Input: part model. Units: mm. Frame: model coordinates. A direction names the side the tool comes from. Give positions to 0.01 mm unless a question says otherwise; leave off trailing zeros. Loops run counter-clockwise (first coordinate to the right, second up) from the corner with the lowest first, then second, coordinate; pieces in that order, holes last. Notation, with made-up numbers: M 63,8 L 98,8 A19 ccw 98,17 Z; hole C 61,60 d6. An arc over 180 degrees is marked long. Use a Markdown table: item, result. Add a question column.
from build123d import *

# Parameters (mm, degrees)
BOSS_EXTRUDE1_DEPTH  = 6.35
SKETCH6_W            = 57.15
SKETCH6_H            = 4.7625
SKETCH6_W_2          = 15.875
CUT_EXTRUDE1_DEPTH   = 85.197384349
M5_CLEARANCE_HOLE1_D = 5.5


with BuildPart() as part:
    # Sketch2 → Boss-Extrude1 (new body)
    with BuildSketch(Plane(origin=(0, 0, 0), x_dir=(1, 0, 0), z_dir=(0, 1, 0))):
        with BuildLine():
            Line((0, 11.1125), (69.85, 11.1125))
            ThreePointArc((69.85, 11.1125), (80.9625, 0), (69.85, -11.1125))
            Line((69.85, -11.1125), (0, -11.1125))
            ThreePointArc((0, -11.1125), (-11.1125, 0), (0, 11.1125))
        make_face()
        with BuildLine():
            Line((15.875, 7.9375), (53.975, 7.9375))
            ThreePointArc((53.975, 7.9375), (61.9125, 0), (53.975, -7.9375))
            Line((53.975, -7.9375), (15.875, -7.9375))
            ThreePointArc((15.875, -7.9375), (7.9375, 0), (15.875, 7.9375))
        make_face(mode=Mode.SUBTRACT)
    extrude(amount=BOSS_EXTRUDE1_DEPTH)

    # Sketch6 → Cut-Extrude1 (cut, through all)
    with BuildSketch(Plane(origin=(0, 0, -11.1125), x_dir=(-1, 0, 0), z_dir=(0, 0, -1))):
        with Locations((-34.925, 2.38125)):
            Rectangle(SKETCH6_W, SKETCH6_H)
        with Locations((-73.025, 3.96875)):
            Rectangle(SKETCH6_W_2, SKETCH6_H)
        with Locations((3.175, 3.96875)):
            Rectangle(SKETCH6_W_2, SKETCH6_H)
    extrude(amount=-CUT_EXTRUDE1_DEPTH, mode=Mode.SUBTRACT)

    # M5 Clearance Hole1 (through all)
    with Locations(Plane(origin=(0, 1.5875, 0), x_dir=(1, 0, 0), z_dir=(0, 1, 0))):
        with Locations((-1.5875, 0), (71.4375, 0)):
            Hole(M5_CLEARANCE_HOLE1_D / 2)


solid = part.part
1) Section query A-A, the plane z = 0. Return the cut outline in (x, y).
2) Section query B-B, the plane y = 3. Return the cut outline in (x, z).
3) Section query D-D, the plane z = -5.75. Return the cut outline in (x, y), and give its area (3 significant figures).
4) Pull-direction query (X, two-part tool) for faces 5 (the cylindrical face through (7.94, 5.55, 0.17)), 6 (the flat face through (70, 0, -3)), 7 (the flat face through (65.088, 4, 0)), 8 (the flat face through (35, 6, 7.938)); classes: pulls with the +X half, pulls with the -X half, needs draft (parallel to the pull), parting line crosses it, or undercut.
5) Section query C-C, the plane x = 39. Return the cut outline in (y, z), and give its area (3 significant figures).
6) Contact query for flat-ended pins moving along their axis: P1, Ø1.4, axis at y = 5, z = 5.5, coming from the +X side; P2, Ø1.4, axis at y = 3, z = -4, coming from the -X side; P3, Ø5, axis at x = 1, z = -0.5, coming from the +Y side; P4, Ø10, axis at x = -0.5, z = 3, coming from the -Y side. Output: stop coordinate, or through.
7) Ray query, line 1 (Z direction, x = 38, y = 5.75); line 2 (X direction, y = 2.5, z = -1.25); line 3 (Y direction, x = 61.5, z = 7.75). Return the intervals inside material, ascending. Write a range as [from, to].
8) Reachability of faces 1 (the flat face through (63.5, 2, 0)), 2 (the cylindrical face through (61.91, 5.55, -0.17)), 3 (the flat face through (75, 1.588, 0)), 4 (the flat face through (4.762, 4, 0)) from +Z, -Z, +X, -X, +Y, -Y: full face, straight path, thin tool, end or side. Return the list, or none.
Entries:
| question | item | result |
|---|---|---|
| 1 | outline | M -11.11,0 L -4.34,0 L -4.34,1.59 L -11.11,1.59 Z; M 1.16,0 L 6.35,0 L 6.35,4.76 L 7.94,4.76 L 7.94,6.35 L 4.76,6.35 L 4.76,1.59 L 1.16,1.59 Z; M 61.91,4.76 L 63.5,4.76 L 63.5,0 L 68.69,0 L 68.69,1.59 L 65.09,1.59 L 65.09,6.35 L 61.91,6.35 Z; M 74.19,0 L 80.96,0 L 80.96,1.59 L 74.19,1.59 Z |
| 2 | outline | M 4.76,-11.11 L 6.35,-11.11 L 6.35,11.11 L 4.76,11.11 Z; M 63.5,-11.11 L 65.09,-11.11 L 65.09,11.11 L 63.5,11.11 Z |
| 3 | outline | M -9.51,0 L 6.35,0 L 6.35,4.76 L 10.4,4.76 L 10.4,6.35 L 4.76,6.35 L 4.76,1.59 L -9.51,1.59 Z; M 59.45,4.76 L 63.5,4.76 L 63.5,0 L 79.36,0 L 79.36,1.59 L 65.09,1.59 L 65.09,6.35 L 59.45,6.35 Z |
| 3 | area | 78.3 mm² |
| 4 | face 5 | undercut |
| 4 | face 6 | needs draft |
| 4 | face 7 | pulls with the +X half |
| 4 | face 8 | undercut |
| 5 | outline | M 4.76,-11.11 L 6.35,-11.11 L 6.35,-7.94 L 4.76,-7.94 Z; M 4.76,7.94 L 6.35,7.94 L 6.35,11.11 L 4.76,11.11 Z |
| 5 | area | 10.1 mm² |
| 6 | P1 | stops at x = 65.09 |
| 6 | P2 | stops at x = 4.76 |
| 6 | P3 | stops at y = 1.59 |
| 6 | P4 | stops at y = 0 |
| 7 | line 1 | z = [-11.11, -7.94], [7.94, 11.11] |
| 7 | line 2 | x = [4.76, 6.35], [63.5, 65.09] |
| 7 | line 3 | y = [4.76, 6.35] |
| 8 | face 1 | +Z, -Z, -Y |
| 8 | face 2 | +Y, -Y |
| 8 | face 3 | +Z, -Z, +X, +Y |
| 8 | face 4 | +Z, -Z, -X, +Y |
